from build123d import *


with BuildPart() as part:
    # Эскиз1 → Повернуть1 (revolve)
    with BuildSketch(Plane(origin=(0, 0, 0), x_dir=(0, 0, -1), z_dir=(1, 0, 0)), mode=Mode.PRIVATE) as revolve_1_sk:
        Polygon((28, 11), (0, 11), (0, 5), (-10, 5), (-10, 3), (2, 3), (2, 8), (23, 8), (23, 10), (28, 10), align=None)
    revolve(revolve_1_sk.sketch.rotate(Axis((0, 0, 28.642974124), (0, 0, -1)), 90), axis=Axis((0, 0, 28.642974124), (0, 0, -1)))


solid = part.part
Model file for the job. Use its own axes, mm. A direction names the side the tool comes from. Round coordinates to 2 decimals unless told otherwise and drop trailing zeros. Order: outer loops, then holes, each group sorted by start corner. A loop starts at its lowest first (then second) coordinate and runs counter-clockwise, first axis right, second up.
(1) Band-saw the part on D-D (x = -9.25). List the corners of the cut face in (y, z).
(2) Pull direction Y, two halves, no side cores. Call faces 1 (the face through (-5, 0, 5)), 2 (the face through (-10, 0, -26)), 3 (the face through (-2, 10, -28)): released by +Y, released by -Y, zero draft, split by the parting line, or undercut.
(3) 3-axis set-ups, long thin cutter, end or side, ignore diameter. For faces 4 (the face through (3.3, -0.1, 10)), 5 (the face through (-3.4, -0.1, -2)), 6 (the face through (2, 5, 0)): which of +Z, -Z, +X, -X, +Y, -Y reach the whole face in a straight line?
(4) Band-saw the part on C-C (z = -8). List the corners of the cut face in (x, y).
(5) Band-saw the part on A-A (x = 0). List the corners of the cut face in (y, z), then the cut area to 3 significant figures.
(6) Drill centre lines: line 1 (Y direction, x = 0, z = -11.75); line 2 (Y direction, x = 0, z = 5.25); line 3 (Z direction, x = -5.75, y = 7.5). Where is each one in solid material? Low to high.
(7) Pin check, flat tips, straight feed: pin 1 (3 mm diameter, centred on x = -1, z = 3, fed in from +Y); pin 2 (7 mm diameter, centred on x = 0, y = 0, fed in from -Z); pin 3 (1 mm diameter, centred on x = 1.5, z = -5.5, fed in from +Y). Stop position of each tip, or through.
Verdict:
1. outline: (-5.95, -28) - (-3.8, -28) - (-3.8, -23) - (3.8, -23) - (3.8, -28) - (5.95, -28) - (5.95, 0) - (-5.95, 0) - close
2. face 1: split by the parting line
2. face 2: undercut
2. face 3: zero draft
3. face 4: +Z, +X, -X, +Y, -Y
3. face 5: -Z
3. face 6: +Z
4. outline: circle Ø22 at (0, 0); hole circle Ø16 at (0, 0)
5. outline: (-11, -28) - (-10, -28) - (-10, -23) - (-8, -23) - (-8, -2) - (-3, -2) - (-3, 10) - (-5, 10) - (-5, 0) - (-11, 0) - close; (3, -2) - (8, -2) - (8, -23) - (10, -23) - (10, -28) - (11, -28) - (11, 0) - (5, 0) - (5, 10) - (3, 10) - close
5. area: 208 mm2
6. line 1: y = -11 to -8, 8 to 11
6. line 2: y = -5 to -3, 3 to 5
6. line 3: z = -23 to 0
7. pin 1: stops at y = 5
7. pin 2: stops at z = -2
7. pin 3: stops at y = 10.95
